Here's how the part is built. I have some questions about the finished solid (model axes, mm). A direction names the side the tool comes from. Coordinates: 2 decimals unless noted, no trailing zeros. Order: outer loops, then holes, each group sorted by start corner. A loop starts at its lowest first (then second) coordinate and runs counter-clockwise, first axis right, second up. Notation, with made-up numbers: (23.5, 43) - (69.5, 43) arc R20 ccw to (69.5, 75) - close; hole circle Ø7 at (12.5, 23.25). An arc over 180 degrees is marked (long way). Answer in a Markdown table with one row per item. Add a question column.
Item 1: On a 3-axis mill with a long thin cutter (end or side, diameter ignored), from which of +Z, -Z, +X, -X, +Y, -Y can I reach the whole of each face in a straight line? I mean faces 1 (the flat face through (-4, -19.5, -4)), 2 (the cylindrical face through (4.01, -1.48, -18.06)), 3 (the cylindrical face through (-7.493, -17.986, 0.33)). Say none if no direction works.
Item 2: Thinking about a two-plate mould opening in Z: for faces 4 (the flat face through (4, 0, 4)), 5 (the cylindrical face through (-6.56, -8.39, -29.53)), 6 (the flat face through (-6, -3, 18)), which applies, +Z half, -Z half, draft (parallel to the pull), parting line (faces both ways), or undercut?
Item 3: I want a section at D-D (y = -5.5). Please give me the cut outline in (x, z), plus the area to 3 significant figures.
Item 4: If I drill on line 1 along Z through (x, y) = (0, -1.75); line 2 along Z through (x, y) = (0, -11); line 3 along X through (y, z) = (-1.25, 15.5), over which ranges is the centre line in solid material (lowest first)? Write a range as from..to.
Item 5: I want a section at C-C (y = -2). Please give me the cut outline in (x, z), plus the area to 3 significant figures.
Item 6: Will these pins go through, and if not, where does the flat tip stop? pin 1 Ø4 at (x, y) = (16.5, -14) entering from +Z; pin 2 Ø5 at (x, y) = (-1.5, -2) entering from -Z; pin 3 Ø2 at (y, z) = (-8.5, 14) entering from -X.
```python
from build123d import *

# Parameters (mm, degrees)
F0_R     = 30.25
F0_R_2   = 5
F1_DEPTH = 17
F2_R     = 7.5
F2_R_2   = 5
F3_DEPTH = 2.5
F4_R     = 21.5
F4_R_2   = 18.5
F5_DEPTH = 3
F6_SIZE  = 0.5


with BuildPart() as f1:
    # F0 (on Front) → F1 (new body)
    with BuildSketch(Plane.XZ):
        Circle(F0_R)
        Circle(F0_R_2, mode=Mode.SUBTRACT)
    extrude(amount=F1_DEPTH)

    # F2 (on face) → F3 (join)
    with BuildSketch(Plane.XZ.offset(17)):
        Circle(F2_R)
        Circle(F2_R_2, mode=Mode.SUBTRACT)
    extrude(amount=F3_DEPTH)

    # F4 (on face) → F5 (cut)
    with BuildSketch(Plane(origin=(0, 0, 0), x_dir=(-1, 0, 0), z_dir=(0, 1, 0))):
        Circle(F4_R)
        Circle(F4_R_2, mode=Mode.SUBTRACT)
    extrude(amount=-F5_DEPTH, mode=Mode.SUBTRACT)

    # F6
    f6_edges = [f1.edges().sort_by_distance(p)[0] for p in [
        (-30.25, -17, 0),
        (-7.5, -19.5, 0),
        (-5, -19.5, 0),
        (-30.25, 0, 0),
        (-5, 0, 0),
    ]]
    chamfer(f6_edges, length=F6_SIZE)


solid = f1.part
```
Values follow:
| question | item | result |
|---|---|---|
| 1 | face 1 | +Z, -Z, +X, -X, -Y |
| 1 | face 2 | +Y |
| 1 | face 3 | -Y |
| 2 | face 4 | draft |
| 2 | face 5 | parting line |
| 2 | face 6 | undercut |
| 3 | outline | circle Ø60.5 at (0, 0); hole circle Ø10 at (0, 0) |
| 3 | area | 2,800 mm^2 |
| 4 | line 1 | z = -30.25..-21.5, -18.5..-5, 5..18.5, 21.5..30.25 |
| 4 | line 2 | z = -30.25..-5, 5..30.25 |
| 4 | line 3 | x = -25.98..-14.9, -10.1..10.1, 14.9..25.98 |
| 5 | outline | circle Ø60.5 at (0, 0); circle Ø37 at (0, 0); hole circle Ø43 at (0, 0); hole circle Ø10 at (0, 0) |
| 5 | area | 2,420 mm^2 |
| 6 | pin 1 | stops at z = 26.55 |
| 6 | pin 2 | stops at z = -30.25 |
| 6 | pin 3 | stops at x = -27.31 |
